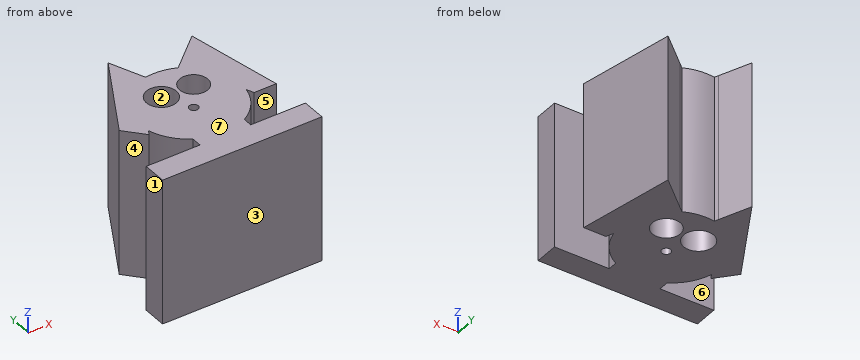
```python
from build123d import *

# Parameters (mm, degrees)
F0_R     = 3.815165
F0_R_2   = 12.72436
F0_R_3   = 11.914866
F1_DEPTH = 61.71997


with BuildPart() as f1:
    # F0 (on Top) → F1 (new body, symmetric)
    with BuildSketch(Plane.XY):
        Polygon((-22.186497, -53.015659), (-54.091621, -53.015659), (-67.938353, -53.015659), (-67.938353, -73.286796), (67.512539, -73.286796), (67.489434, -53.015659), (20.967111, -53.015659), align=None)
        with BuildLine():
            Line((-22.186497, -44.352168), (-22.186497, -53.015659))
            Line((-22.186497, -53.015659), (20.967111, -53.015659))
            Line((20.967111, -53.015659), (20.967111, -45.047))
            ThreePointArc((20.967111, -45.047), (-0.701729, -50.415619), (-22.186497, -44.352168))
        make_face()
        with BuildLine():
            ThreePointArc((-42.052504, -18.299424), (-34.660477, -33.263368), (-22.186497, -44.352168))
            ThreePointArc((-22.186497, -44.352168), (-0.701729, -50.415619), (20.967111, -45.047))
            ThreePointArc((20.967111, -45.047), (34.948374, -32.881486), (42.611378, -16.006836))
            ThreePointArc((42.611378, -16.006836), (43.342832, -11.446167), (43.587566, -6.833702))
            ThreePointArc((43.587566, -6.833702), (38.545513, 13.516219), (24.585849, 29.158129))
            ThreePointArc((24.585849, 29.158129), (21.489345, 31.088375), (18.242246, 32.752865))
            ThreePointArc((18.242246, 32.752865), (5.862878, 36.357761), (-7.029507, 36.183293))
            ThreePointArc((-7.029507, 36.183293), (-8.799871, 35.856322), (-10.555224, 35.456523))
            ThreePointArc((-10.555224, 35.456523), (-37.607429, 15.201659), (-42.052504, -18.299424))
        make_face()
        with Locations((0, -13.019726)):
            Circle(F0_R, mode=Mode.SUBTRACT)
        with Locations((-11.483821, 10.258501)):
            Circle(F0_R_2, mode=Mode.SUBTRACT)
        with Locations((15.761618, 9.937936)):
            Circle(F0_R_3, mode=Mode.SUBTRACT)
        with BuildLine():
            Line((-44.51011, -22.493784), (-42.052504, -18.299424))
            ThreePointArc((-42.052504, -18.299424), (-37.607429, 15.201659), (-10.555224, 35.456523))
            Line((-10.555224, 35.456523), (-8.289508, 39.323387))
            Line((-8.289508, 39.323387), (-18.786313, 65.482855))
            Line((-18.786313, 65.482855), (-58.853593, -6.507952))
            Line((-58.853593, -6.507952), (-44.51011, -22.493784))
        make_face()
        with BuildLine():
            ThreePointArc((43.587566, -6.833702), (43.342832, -11.446167), (42.611378, -16.006836))
            Line((42.611378, -16.006836), (45.060731, -22.143964))
            Line((45.060731, -22.143964), (63.954249, -22.143964))
            Line((63.954249, -22.143964), (48.082457, 58.999361))
            Line((48.082457, 58.999361), (21.875692, 35.948728))
            Line((21.875692, 35.948728), (24.585849, 29.158129))
            ThreePointArc((24.585849, 29.158129), (38.545513, 13.516219), (43.587566, -6.833702))
        make_face()
        with BuildLine():
            Line((-8.289508, 39.323387), (-10.555224, 35.456523))
            ThreePointArc((-10.555224, 35.456523), (-8.799871, 35.856322), (-7.029507, 36.183293))
            Line((-7.029507, 36.183293), (-8.289508, 39.323387))
        make_face()
        with BuildLine():
            ThreePointArc((18.242246, 32.752865), (21.489345, 31.088375), (24.585849, 29.158129))
            Line((24.585849, 29.158129), (21.875692, 35.948728))
            Line((21.875692, 35.948728), (18.242246, 32.752865))
        make_face()
    extrude(amount=F1_DEPTH, both=True)


solid = f1.part
```
CAD build for the part. Positions are in the model's coordinates, mm. Face numbers are marked on the shaded views. A direction names the side the tool comes from. Coordinates: 2 decimals unless noted, no trailing zeros. Order: outer loops, then holes, each group sorted by start corner. A loop starts at its lowest first (then second) coordinate and runs counter-clockwise, first axis right, second up. Notation, with made-up numbers: M 5,6 L 48,6 A28 cw 48,27 Z; hole C 30,28 d10. An arc over 180 degrees is marked long. Write each question's results on one line, items separated by ' | '. Start each with the question number.
Q1. Flat gauge pins, fed straight in: P1, Ø14, axis at x = 33, z = -16, coming from the +Y side; P2, Ø4.5, axis at x = 0, y = -13.02, coming from the -Z side; P3, Ø6, axis at y = -21.5, z = -24.5, coming from the +X side; P4, Ø1.5, axis at x = -32.5, z = 11, coming from the +Y side. Where does each tip first touch, or does it go through?
Q2. Which spindle directions (+Z, -Z, +X, -X, +Y, -Y) get a long thin tool onto all of the face, cutting with end or side? Do the marked faces 5, 6 and 7. Say none if no direction does.
Q3. Cut at D-D (y = 29.5). List the corners of the cut face in (x, z), then the cut area to 3 significant figures.
Q4. Cut at A-A (x = 50.5). List the corners of the cut face in (y, z), then the cut area to 3 significant figures.
Q5. Pull direction Y, two halves, no side cores. Call the marked faces 1, 2, 3 and 4: +Y half, -Y half, draft (parallel to the pull), parting line (faces both ways), or undercut.
Q6. Cut at C-C (x = -50.5). List the corners of the cut face in (y, z), then the cut area to 3 significant figures.
Q7. Cut at B-B (z = 11). List the corners of the cut face in (x, y), then the cut area to 3 significant figures.
Q8. Drill centre lines: probe 1 along Y at (x, z) = (0, 9); probe 2 along X at (y, z) = (20, 40); probe 3 along X at (y, z) = (-14, -12). Where is each one in solid material? Low to high. Write a range as from..to.
Found:
1) P1: y = 51.89 | P2: through | P3: x = 63.95 | P4: y = 42.19
2) face 5: +Z, -Z, +X | face 6: +Z, -Z, -X | face 7: +Z, +X, -X, +Y, -Y
3) outline: M -38.81,-61.72 L 53.85,-61.72 L 53.85,61.72 L -38.81,61.72 Z | area: 11,400 mm²
4) outline: M -73.29,-61.72 L -53.02,-61.72 L -53.02,61.72 L -73.29,61.72 Z; M -22.14,-61.72 L 46.64,-61.72 L 46.64,61.72 L -22.14,61.72 Z | area: 11,000 mm²
5) face 1: draft | face 2: undercut | face 3: -Y half | face 4: undercut
6) outline: M -73.29,-61.72 L -53.02,-61.72 L -53.02,61.72 L -73.29,61.72 Z; M -15.82,-61.72 L 8.5,-61.72 L 8.5,61.72 L -15.82,61.72 Z | area: 5,500 mm²
7) outline: M -67.94,-73.29 L 67.51,-73.29 L 67.49,-53.02 L 20.97,-53.02 L 20.97,-45.05 A43.59 ccw 42.61,-16.01 L 45.06,-22.14 L 63.95,-22.14 L 48.08,59 L 18.24,32.75 A43.59 ccw -7.03,36.18 L -18.79,65.48 L -58.85,-6.51 L -44.51,-22.49 L -42.05,-18.3 A43.59 ccw -22.19,-44.35 L -22.19,-53.02 L -67.94,-53.02 Z; hole C -11.48,10.26 d25.45; hole C 0,-13.02 d7.63; hole C 15.76,9.94 d23.83 | area: 10,500 mm²
8) probe 1: -73.29..-16.83, -9.2..4.78, 15.74..36.75 | probe 2: -44.1..-19.67, -3.3..9.38, 22.14..55.71 | probe 3: -52.13..-3.69, 3.69..62.36
